Autodesk Inventor part; units mm, degrees
ref_plane "YZ Plane" through (0, 0, 0) normal (1, 0, 0) x (0, 1, 0)
ref_plane "XZ Plane" through (0, 0, 0) normal (0, 1, 0) x (-1, 0, 0)
ref_plane "XY Plane" through (0, 0, 0) normal (0, 0, 1) x (1, 0, 0)
sketch "Sketch1" plane through (0, 0, 0) normal (0, 1, 0) x (-1, 0, 0)
  circle A0 centre (0, 0) radius 11.43
  circle A1 centre (0, 0) radius 9.525
  dimension "d0" = 22.86
  dimension "d1" = 19.05
extrude "Extrusion1" add sketch "Sketch1" along normal blind 6.35
sketch "Sketch2" plane through (0, 6.35, 0) normal (0, 1, 0) x (1, 0, 0)
  circle A0 centre (0, 0) radius 11.43
extrude "Extrusion2" add sketch "Sketch2" along normal blind 3.175
sketch "Sketch3" plane through (0, 9.525, 0) normal (0, 1, 0) x (1, 0, 0)
  circle A0 centre (0, 0) radius 1.1
  dimension "d6" = 2.2
extrude "Extrusion3" cut sketch "Sketch3" against normal blind 7.9375
sketch "Sketch6" plane through (0, 0, 0) normal (0, -1, 0) x (1, 0, 0)
  line L0 (-16.0948, 0) -> (0, 0)
  line L1 (0, 0) -> (0, -15.3841)
  line L2 (0, -15.3841) -> (-16.0948, -15.3841)
  line L3 (-16.0948, -15.3841) -> (-16.0948, 0)
  line L4 (-16.0948, 14.6504) -> (12.3807, 14.6504)
  line L5 (12.3807, 14.6504) -> (12.3807, -15.3841)
  line L6 (12.3807, -15.3841) -> (-16.0948, -15.3841)
  line L7 (-16.0948, -15.3841) -> (-16.0948, 14.6504)
extrude "Extrusion6" cut sketch "Sketch6" against normal blind 6.35 contours L7 L4 L5 L6 L1 L0
sketch "Sketch7" plane through (0, 0, -9.525) normal (1, 0, 0) x (0, 0, -1)
  line L0 (1.905, 6.35) -> (-20.955, 6.35)
  line L1 (1.905, 6.35) -> (0, 6.35)
  line L2 (0, 6.35) -> (0, 0)
  line L3 (0, 0) -> (1.905, 0)
  line L4 (1.905, 0) -> (1.905, 6.35)
  point P0 (-9.525, 0)
  point P1 (-9.525, 6.35)
extrude "Extrusion7" add sketch "Sketch7" along normal blind 11.43
sketch "Sketch16" plane through (0, 0, 0) normal (0, -1, 0) x (1, 0, 0)
  point P0 (0, 0)
sketch "Sketch17" plane through (-11.43, 0, 0) normal (0, 0, 1) x (1, 0, 0)
  line L0 (0, 0) -> (0, 6.35)
  line L1 (0, 6.35) -> (1.9041, 6.35)
  line L2 (1.9041, 6.35) -> (1.9041, 0)
  line L3 (1.9041, 0) -> (0, 0)
  line L4 (0, 0) -> (0, 6.35)
  point P0 (11.43, 0)
extrude "Extrusion16" add sketch "Sketch17" along normal blind 12.7
sketch "Sketch18" plane through (0, 6.35, 0) normal (0, -1, 0) x (1, 0, 0)
  circle A0 centre (0, 0) radius 1.1
  line L0 (0, 0) -> (-18.4871, -7.6576)
  line L1 (0, 0) -> (20.0102, 0) construction
  line L2 (-18.4871, -7.6576) -> (1.1, -41.4972)
  line L3 (1.1, -41.4972) -> (21.3747, 0)
  line L4 (21.3747, 0) -> (0, 0)
  dimension "d61" = 157.5
extrude "Extrusion17" cut sketch "Sketch18" along normal blind 25.4 contours L4 L3 L2 L0 A0 | A0 L0 L4 picked at (-0.5236, -0.5052)
sketch "Sketch21" plane through (0, 9.525, 0) normal (0, 1, 0) x (1, 0, 0)
  line L0 (0, 0) -> (76.2, 0) construction
  circle A0 centre (0, 0) radius 11.43
  line L1 (8.0168, -8.1472) -> (33.4168, -8.1472)
  line L2 (8.0168, -8.1472) -> (33.4168, -8.1472) construction
  circle A1 centre (53.8815, -53.8815) radius 10.16
  line L3 (33.4168, -8.1472) -> (46.6973, -46.6973)
  line L4 (8.0822, 8.0822) -> (38.5622, 8.0822)
  line L5 (53.8815, -53.8815) -> (61.0657, -46.6973)
  line L6 (53.8815, -53.8815) -> (64.0415, -53.8815) construction
  line L7 (61.0657, -46.6973) -> (38.5622, 8.0822)
  line L8 (0, 0) -> (8.0168, -8.1472)
  line L9 (46.6973, -46.6973) -> (53.8815, -53.8815)
  line L10 (8.0168, 8.1472) -> (8.0168, -8.1472)
  dimension "d85" = 25.4
  dimension "d86" = 0
  dimension "d87" = 20.32
  dimension "d88" = 30.48
  dimension "d89" = 45
extrude "Extrusion20" add sketch "Sketch21" against normal blind 3.175 contours L5 L9 A1 | A1 L9 L5
sketch "Sketch22" plane through (0, 9.525, 0) normal (0, 1, 0) x (1, 0, 0)
  circle A0 centre (0, 0) radius 1.1
  line L0 (0, 0) -> (8.0822, 8.0822)
  circle A1 centre (0, 0) radius 11.43
  line L1 (0, 0) -> (11.43, 0) construction
  line L2 (8.0822, 8.0822) -> (39.8322, 8.0822)
  line L3 (39.8322, 8.0822) -> (53.8815, -43.7215)
  circle A2 centre (53.8815, -53.8815) radius 10.16
  line L4 (0, 0) -> (8.0822, -8.0822)
  line L5 (8.0822, -8.0822) -> (33.4822, -8.0822)
  line L6 (33.4822, -8.0822) -> (43.7215, -53.8815)
  line L7 (53.8815, -43.7215) -> (43.7215, -53.8815)
  dimension "d92" = 45
  dimension "d93" = 31.75
  dimension "d94" = 25.4
extrude "Extrusion21" add sketch "Sketch22" against normal blind 3.175 contours L2 L3 A2 L6 L5 A1
fillet "Fillet6" radius 25.4 1 edges at (33.4822, 7.9375, 8.0822)
fillet "Fillet7" radius 50.8 1 edges at (39.8322, 7.9375, -8.0822)
For this review, take the finished solid that the model builds, in its own axes (mm). A direction names the side the tool comes from. Coordinates: 2 decimals unless noted, no trailing zeros. Write each loop counter-clockwise with the first axis right and the second up, starting at its lowest first coordinate (ties: lowest second). Pieces come first, ordered by that corner, then holes.
(1) Tool access review of faces 1 (the face through (35, 9.525, 18)), 2 (the face through (-10, 6.35, 8)), 3 (the face through (-9.526, 3, 6)), 4 (the face through (-9.668, 3.219, -4.004)), 5 (the face through (28.83, 7.92, 13.51)): name each direction out of +Z, -Z, +X, -X, +Y, -Y from which nothing blocks a thin tool from reaching the whole face with its end or side.
(2) Add section C-C on z = 4.5. Give the boundary of the cut face in (x, y) (3 decimals).
(3) Add section D-D on x = 51.5. Give the boundary of the cut face in (y, z) (3 decimals).
(4) Add section A-A on x = 0. Give the boundary of the cut face in (y, z) (3 decimals), then the cut area to 3 significant figures.
(5) For pin 1 Ø12 at (x, z) = (26, 28) entering from -Y; pin 2 Ø3 at (y, z) = (4, 5) entering from +X; pin 3 Ø1 at (x, y) = (-10, 2) entering from +Z; pin 4 Ø1.5 at (x, y) = (39.5, 6) entering from -Z, all flat-tipped, find the tip position at first contact; note any pin that passes through.
(6) Add section B-B on y = 7.5. Give the boundary of the cut face in (x, z).
(7) Wall thickness on probe 1 along Z at (x, y) = (0, 7.9); probe 2 along X at (y, z) = (8.65, 0); probe 3 along Y at (x, z) = (10.5, 0.5) (3 decimals): over which ranges is each line inside the solid? List them lowest first.
(8) The part is to be moulded in two halves that separate along X. For faces 6 (the face through (32, 6.35, 15)), 7 (the face through (60.825, 7.96, 61.299)), 8 (the face through (11, 8, 8.082)), 9 (the face through (1.05, 7.96, -0.33)), say which applies: +X half, -X half, draft (parallel to the pull), parting line (faces both ways), or undercut.
Answer sheet:
1. face 1: +Z, -Z, +X, -X, +Y
1. face 2: +Z, -X, +Y
1. face 3: +Z, +X, -Y
1. face 4: -Z, +X, -Y
1. face 5: +Z, +Y, -Y
2. outline: (-11.43, 0) - (-9.526, 0) - (-9.526, 6.35) - (34.885, 6.35) - (34.885, 9.525) - (-10.507, 9.525) - (-10.507, 6.35) - (-11.43, 6.35) - close
3. outline: (6.35, 34.94) - (9.525, 34.94) - (9.525, 63.758) - (6.35, 63.758) - close
4. outline: (6.35, -11.43) - (9.525, -11.43) - (9.525, -1.1) - (6.35, -1.1) - close; (6.35, 1.1) - (9.525, 1.1) - (9.525, 11.43) - (6.35, 11.43) - close
4. area: 65.6 mm2
5. pin 1: passes through
5. pin 2: stops at x = -9.53
5. pin 3: stops at z = 12.7
5. pin 4: stops at z = 8.49
6. outline: (8.08, -8.08) arc R50.8 ccw to (49.86, 28.9) - (53.88, 43.72) arc R10.16 ccw (long way) to (43.72, 53.88) - (37.92, 27.94) arc R25.4 cw to (13.13, 8.08) - (8.08, 8.08) arc R11.43 ccw (long way) to start; hole circle Ø2.2 at (0, 0)
7. probe 1: z = -11.43 to -1.1, 1.1 to 11.43
7. probe 2: x = -11.43 to -1.1, 1.1 to 29.12
7. probe 3: y = 6.35 to 9.525
8. face 6: draft
8. face 7: parting line
8. face 8: undercut
8. face 9: undercut
